Build history of the part. All positions in model axes, mm. A direction names the side the tool comes from. Coordinates: 2 decimals unless noted, no trailing zeros. Loops run counter-clockwise (first coordinate to the right, second up) from the corner with the lowest first, then second, coordinate; pieces in that order, holes last.
Item 1: Drill centre lines: line 1 along X through (y, z) = (7, -132.5); line 2 along X through (y, z) = (6.5, -140.5); line 3 along X through (y, z) = (8.25, -144). Where is each one in solid material? Low to high.
Item 2: Flat gauge pins, fed straight in: pin 1 (2.5 mm diameter, centred on x = 0, z = 15.5, fed in from -Y); pin 2 (6 mm diameter, centred on y = 3.5, z = -13.5, fed in from -X); pin 3 (5 mm diameter, centred on x = -1.5, y = 3.5, fed in from +Z); pin 4 (5 mm diameter, centred on x = 3, y = 2.5, fed in from -Z). Where does each tip first touch, or does it go through?
Item 3: Cut at A-A (x = 0). List the corners of the cut face in (y, z), and give its area (3 significant figures).
Item 4: Mould opens along X. For faces 4 (the face through (-50.596, 4.93, 20.04)), 5 (the face through (56.63, 4.93, -150.54)), 6 (the face through (0, 5, 0)) say: released by +X, released by -X, zero draft, split by the parting line, or undercut.
Item 5: Cut at C-C (z = -28). List the corners of the cut face in (x, y).
Item 6: Cut at B-B (z = 15.5). List the corners of the cut face in (x, y), and give its area (3 significant figures).
Item 7: 3-axis set-ups, long thin cutter, end or side, ignore diameter. For faces 1 (the face through (44.283, 4.93, -149.498)), 2 (the face through (-38.893, 4.93, -134.608)), 3 (the face through (-81.855, 4.93, -33.768)): which of +Z, -Z, +X, -X, +Y, -Y reach the whole face in a straight line?
Item 8: Cut at D-D (y = 1.5). Count the separate pieces of the cut face and the enclosed holes in it, and give its area (3 significant figures).
from build123d import *

# Parameters (mm, degrees)
EXTRUDE_1_DEPTH     = 10
CUT_EXTRUDE_1_REACH = 193.071
SKETCH_2_R          = 2.15
FILLET_1_R          = 1


with BuildPart() as part:
    # 草图1 → 凸台-拉伸1 (new body)
    with BuildSketch(Plane(origin=(0, 0, 0), x_dir=(1, 0, 0), z_dir=(0, 1, 0))):
        with BuildLine():
            Line((-23, 0), (23, 0))
            Line((23, 0), (50.285797586, 32.5179473))
            ThreePointArc((50.285797586, 32.5179473), (50.973364459, 33.797571478), (51.093655637, 35.245230373))
            Line((51.093655637, 35.245230373), (36.048986901, 157.774224452))
            ThreePointArc((36.048986901, 157.774224452), (37.845835898, 160.483359772), (40.800128771, 159.126807481))
            ThreePointArc((40.800128771, 159.126807481), (44.320748104, 149.357169855), (46.104078009, 139.126807481))
            ThreePointArc((46.104078009, 139.126807481), (49.378558351, 136.397919911), (52.076572947, 139.697884476))
            Line((52.076572947, 139.697884476), (50.986595809, 150.068324212))
            ThreePointArc((50.986595809, 150.068324212), (51.871765629, 151.945152782), (53.94525884, 152.026620552))
            Line((53.94525884, 152.026620552), (59.390134233, 149.008476838))
            ThreePointArc((59.390134233, 149.008476838), (60.038548982, 148.434807928), (60.38376936, 147.640855414))
            Line((60.38376936, 147.640855414), (81.817064827, 37.376109146))
            ThreePointArc((81.817064827, 37.376109146), (81.863649007, 33.817543133), (80.66104703, 30.468019192))
            Line((80.66104703, 30.468019192), (47.934130885, -26.216662346))
            ThreePointArc((47.934130885, -26.216662346), (46.628637115, -27.522156116), (44.845299462, -28))
            Line((44.845299462, -28), (10.707106781, -28))
            ThreePointArc((10.707106781, -28), (10.515765065, -27.961939766), (10.353553391, -27.853553391))
            Line((10.353553391, -27.853553391), (10, -27.5))
            Line((10, -27.5), (-10, -27.5))
            Line((-10, -27.5), (-10.353553391, -27.853553391))
            ThreePointArc((-10.353553391, -27.853553391), (-10.515765065, -27.961939766), (-10.707106781, -28))
            Line((-10.707106781, -28), (-44.845299462, -28))
            ThreePointArc((-44.845299462, -28), (-45.845299462, -27.732050808), (-46.577350269, -27))
            Line((-46.577350269, -27), (-54.72793721, -12.882769307))
            Line((-54.72793721, -12.882769307), (-80.66104703, 30.468019192))
            ThreePointArc((-80.66104703, 30.468019192), (-81.863649007, 33.817543133), (-81.817064827, 37.376109146))
            Line((-81.817064827, 37.376109146), (-60.205817968, 148.556335961))
            ThreePointArc((-60.205817968, 148.556335961), (-55.396009288, 161.24228741), (-46.622387315, 171.590774314))
            ThreePointArc((-46.622387315, 171.590774314), (-43.239620762, 171.913395421), (-41.72575767, 168.871124481))
            ThreePointArc((-41.72575767, 168.871124481), (-41.549863048, 156.552194932), (-37.633288365, 144.871124481))
            Line((-37.633288365, 144.871124481), (-51.176674229, 34.569098196))
            ThreePointArc((-51.176674229, 34.569098196), (-51.109221395, 33.75732882), (-50.723670812, 33.03978429))
            Line((-50.723670812, 33.03978429), (-23, 0))
        make_face()
    extrude(amount=EXTRUDE_1_DEPTH)

    # 草图2 → 切除-拉伸1 (cut, up to next)
    with BuildSketch(Plane(origin=(0, 10, 0), x_dir=(1, 0, 0), z_dir=(0, 1, 0)), mode=Mode.PRIVATE) as cut_extrude_1_sk1:
        with Locations(Location((0, -23.5, 0), (0, 0, 270))):
            Circle(SKETCH_2_R)
    cut_extrude_1_tool1 = extrude(cut_extrude_1_sk1.sketch, amount=-CUT_EXTRUDE_1_REACH, mode=Mode.PRIVATE) & part.part
    # 草图2 → 切除-拉伸1 (cut, up to next)
    with BuildSketch(Plane(origin=(0, 10, 0), x_dir=(1, 0, 0), z_dir=(0, 1, 0)), mode=Mode.PRIVATE) as cut_extrude_1_sk2:
        with Locations(Location((0, -15.5, 0), (0, 0, 270))):
            Circle(SKETCH_2_R)
    cut_extrude_1_tool2 = extrude(cut_extrude_1_sk2.sketch, amount=-CUT_EXTRUDE_1_REACH, mode=Mode.PRIVATE) & part.part
    # 草图2 → 切除-拉伸1 (cut, up to next)
    with BuildSketch(Plane(origin=(0, 10, 0), x_dir=(1, 0, 0), z_dir=(0, 1, 0)), mode=Mode.PRIVATE) as cut_extrude_1_sk3:
        with BuildLine():
            Line((-40.580117827, 120.871124481), (-43.035809045, 100.871124481))
            ThreePointArc((-43.035809045, 100.871124481), (-49.262696908, 118.999215044), (-50.998704156, 138.08816679))
            ThreePointArc((-50.998704156, 138.08816679), (-47.997070546, 140.99999857), (-45.001129375, 138.082310248))
            ThreePointArc((-45.001129375, 138.082310248), (-43.758467402, 129.228108775), (-40.580117827, 120.871124481))
        make_face()
    cut_extrude_1_tool3 = extrude(cut_extrude_1_sk3.sketch, amount=-CUT_EXTRUDE_1_REACH, mode=Mode.PRIVATE) & part.part
    add(cut_extrude_1_tool1.solids().sort_by_distance((0, 10, 23.5))[0], mode=Mode.SUBTRACT)
    add(cut_extrude_1_tool2.solids().sort_by_distance((0, 10, 15.5))[0], mode=Mode.SUBTRACT)
    add(cut_extrude_1_tool3.solids().sort_by_distance((-46.028937, 10, -123.122257))[0], mode=Mode.SUBTRACT)

    # 圆角1
    fillet_1_edges = [part.edges().sort_by_distance(p)[0] for p in [
        (-40.580117827, 5, -120.871124481),
        (-37.633288365, 5, -144.871124481),
    ]]
    fillet(fillet_1_edges, radius=FILLET_1_R)


solid = part.part
Filled sheet:
1. line 1: x = -63.33 to -50.97, -44.45 to -39.15, 39.15 to 63.33
1. line 2: x = -61.77 to -49.66, -46.34 to -38.17, 38.17 to 45.97, 51.99 to 61.77
1. line 3: x = -61.09 to -37.74, 37.74 to 45.48, 51.62 to 61.09
2. pin 1: passes through
2. pin 2: stops at x = -72.31
2. pin 3: stops at z = 27.5
2. pin 4: stops at z = 0
3. outline: (0, 0) - (10, 0) - (10, 13.35) - (0, 13.35) - close; (0, 17.65) - (10, 17.65) - (10, 21.35) - (0, 21.35) - close; (0, 25.65) - (10, 25.65) - (10, 27.5) - (0, 27.5) - close
3. area: 189 mm2
4. face 4: released by -X
4. face 5: released by +X
4. face 6: undercut
5. outline: (-79.18, 0) - (-46.49, 0) - (-46.49, 10) - (-79.18, 10) - close; (46.49, 0) - (79.24, 0) - (79.24, 10) - (46.49, 10) - close
6. outline: (-53.22, 0) - (-2.15, 0) - (-2.15, 10) - (-53.22, 10) - close; (2.15, 0) - (54.12, 0) - (54.12, 10) - (2.15, 10) - close
6. area: 1,030 mm2
7. face 1: -Z, +Y, -Y
7. face 2: +Y, -Y
7. face 3: -X, +Y, -Y
8. separate pieces: 1
8. enclosed holes: 2
8. area: 11,700 mm2
